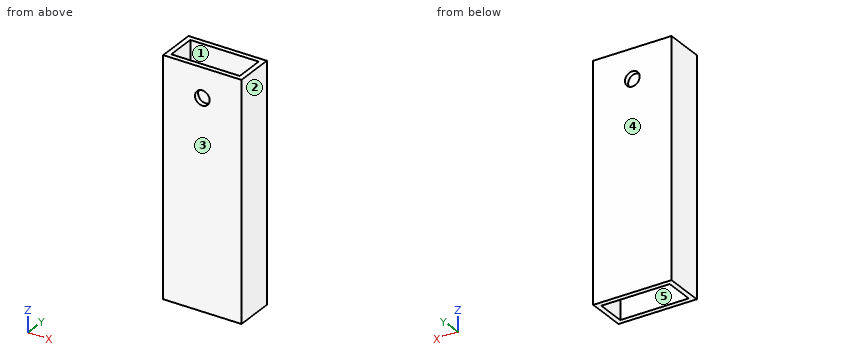
from build123d import *

# Parameters (mm, degrees)
SKETCH1_W           = 50.8
SKETCH1_H           = 25.4
SKETCH1_W_2         = 44.45
SKETCH1_H_2         = 19.05
BOSS_EXTRUDE1_DEPTH = 152.4
SKETCH2_R           = 4.7625
CUT_EXTRUDE1_DEPTH  = 157.576115675


with BuildPart() as part:
    # Sketch1 → Boss-Extrude1 (new body)
    with BuildSketch(Plane.XY):
        Rectangle(SKETCH1_W, SKETCH1_H)
        Rectangle(SKETCH1_W_2, SKETCH1_H_2, mode=Mode.SUBTRACT)
    extrude(amount=BOSS_EXTRUDE1_DEPTH)

    # Sketch2 → Cut-Extrude1 (cut, through all)
    with BuildSketch(Plane(origin=(0, 12.7, 0), x_dir=(1, 0, 0), z_dir=(0, 1, 0))):
        with Locations(Location((0, -133.35, 0), (0, 0, 270))):
            Circle(SKETCH2_R)
    extrude(amount=-CUT_EXTRUDE1_DEPTH, mode=Mode.SUBTRACT)


solid = part.part
Can you work these out from the model? Positions are in its coordinate system, mm. Face numbers are marked on the shaded views. A direction names the side the tool comes from. Give positions to 0.01 mm unless a question says otherwise; leave off trailing zeros. Order: outer loops, then holes, each group sorted by start corner. A loop starts at its lowest first (then second) coordinate and runs counter-clockwise, first axis right, second up. Notation, with made-up numbers: M 39.25,-28.75 L 93.25,-28.75 A23 cw 93.25,-14.75 Z; hole C -17,54.5 d1. An arc over 180 degrees is marked long. Use a Markdown table: item, result. Add a question column.
Item 1: For the marked faces 4 and 5, which set-ups out of +Z, -Z, +X, -X, +Y, -Y let a thin tool reach every point of the face, with its end or its side?
Item 2: Suppose I cut it at D-D (y = 5.25). List the corners of the cut face in (x, z) for me (3 decimals), then the cut area to 3 significant figures.
Item 3: Suppose I cut it at A-A (x = 0). List the corners of the cut face in (y, z) for me (1 decimal), then the cut area to 3 significant figures.
Item 4: Suppose I cut it at C-C (x = 19.5). List the corners of the cut face in (y, z) for me (3 decimals).
Item 5: We'd pull the mould along Y, two halves only. Please class the marked faces 1, 2 and 3: +Y half, -Y half, draft (parallel to the pull), parting line (faces both ways), or undercut.
Item 6: Will this pin go through, and if not, where does the flat tip stop? pin 1 (11 mm diameter, centred on x = 0, z = 133.35, fed in from -Y).
Item 7: Suppose I cut it at B-B (z = 133.35). List the corners of the cut face in (x, y) for me (1 decimal).
Item 8: If I drill on L1, parallel to Y at x = -4, z = 65 (3 decimals); L2, parallel to X at y = -5, z = 83.5 (3 decimals); L3, parallel to X at y = -10.7, z = 133.35, over which ranges is the centre line in solid material (lowest first)? Write a range as [from, to].
Answer sheet:
| question | item | result |
|---|---|---|
| 1 | face 4 | +Z, -Z, +X, -X, +Y |
| 1 | face 5 | +Z, -Z |
| 2 | outline | M -25.4,0 L -22.225,0 L -22.225,152.4 L -25.4,152.4 Z; M 22.225,0 L 25.4,0 L 25.4,152.4 L 22.225,152.4 Z |
| 2 | area | 968 mm² |
| 3 | outline | M -12.7,0 L -9.5,0 L -9.5,128.6 L -12.7,128.6 Z; M -12.7,138.1 L -9.5,138.1 L -9.5,152.4 L -12.7,152.4 Z; M 9.5,0 L 12.7,0 L 12.7,128.6 L 9.5,128.6 Z; M 9.5,138.1 L 12.7,138.1 L 12.7,152.4 L 9.5,152.4 Z |
| 3 | area | 907 mm² |
| 4 | outline | M -12.7,0 L -9.525,0 L -9.525,152.4 L -12.7,152.4 Z; M 9.525,0 L 12.7,0 L 12.7,152.4 L 9.525,152.4 Z |
| 5 | face 1 | undercut |
| 5 | face 2 | draft |
| 5 | face 3 | -Y half |
| 6 | pin 1 | stops at y = -12.7 |
| 7 | outline | M -25.4,-12.7 L -4.8,-12.7 L -4.8,-9.5 L -22.2,-9.5 L -22.2,9.5 L -4.8,9.5 L -4.8,12.7 L -25.4,12.7 Z; M 4.8,-12.7 L 25.4,-12.7 L 25.4,12.7 L 4.8,12.7 L 4.8,9.5 L 22.2,9.5 L 22.2,-9.5 L 4.8,-9.5 Z |
| 8 | L1 | y = [-12.7, -9.525], [9.525, 12.7] |
| 8 | L2 | x = [-25.4, -22.225], [22.225, 25.4] |
| 8 | L3 | x = [-25.4, -4.76], [4.76, 25.4] |
